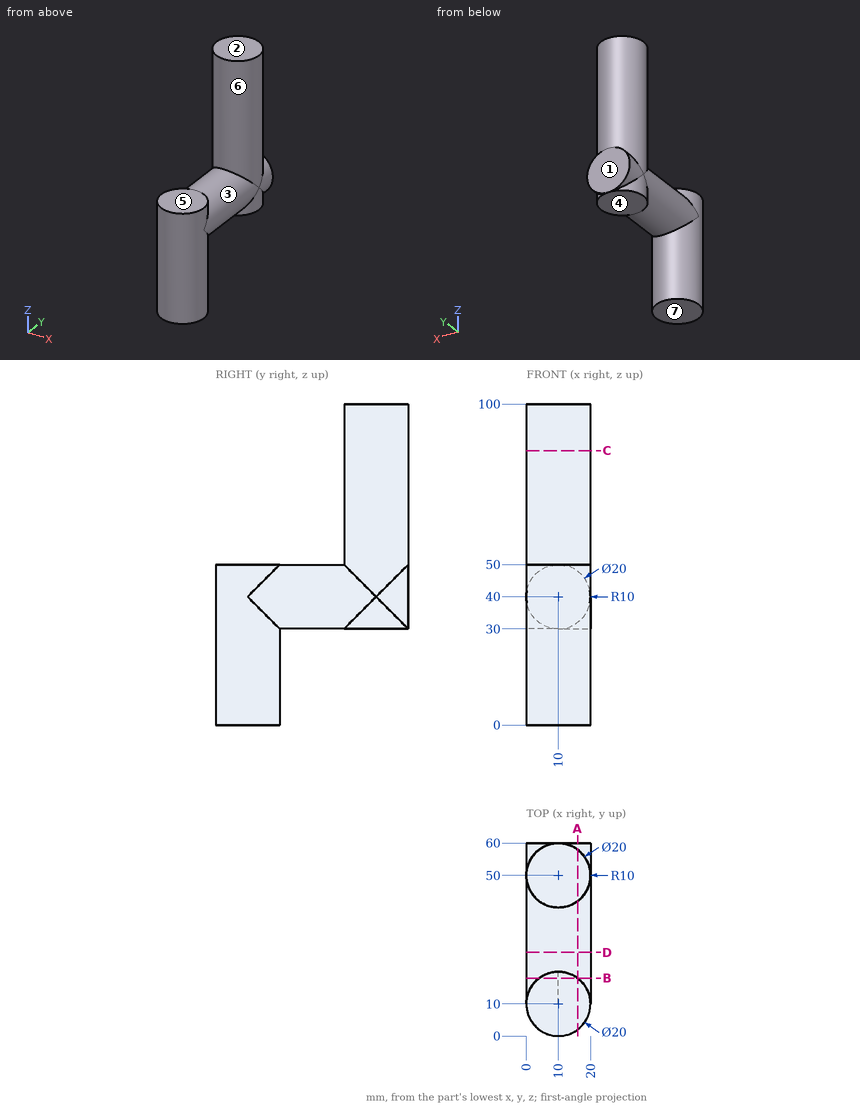
Check sheet for the drawn part. Datum: minimum x, y, z corner. Units: mm. A direction names the side the tool comes from. Coordinates: 2 decimals unless noted, no trailing zeros. Order: outer loops, then holes, each group sorted by start corner. A loop starts at its lowest first (then second) coordinate and runs counter-clockwise, first axis right, second up. Notation, with made-up numbers: M -16,-36 L 11,-36 A21 ccw 11,-14 Z; hole C -36,17 d3. An arc over 180 degrees is marked long. One line per item, written item: value. Start each with the question number.
Item 1: Mould release check, pull along Y, two halves, no side actions. Record for the marked faces 1, 2 and 3: released by +Y, released by -Y, zero draft, split by the parting line, or undercut.
Item 2: Sectioned sample at D-D (y = 26). Enter the section's corners in (x, z), then the cut area to 3 significant figures.
Item 3: Sectioned sample at C-C (z = 85.5). Enter the section's corners in (x, y).
Item 4: Sectioned sample at A-A (x = 16). Enter the section's corners in (y, z), then the cut area to 3 significant figures.
Item 5: Access from +Z, -Z, +X, -X, +Y, -Y to the whole of each face (thin tool, end or side, straight path). Record for the marked faces 4, 5, 6 and 7.
Item 6: Sectioned sample at B-B (y = 18). Enter the section's corners in (x, z).
Item 7: Scan lines: probe 1 along Z at (x, y) = (2.25, 45.5); probe 2 along Z at (x, y) = (14.75, 13.5); probe 3 along X at (y, z) = (4, 8). Record each from-to range of solid material in increasing order.
Item 8: Gauge pin test, flat ends, axial feed: pin 1 (6 mm diameter, centred on x = 11.5, y = 7, fed in from +Z); pin 2 (3 mm diameter, centred on x = 12, z = 69.5, fed in from -Y); pin 3 (1 mm diameter, centred on y = 47.5, z = 50.5, fed in from -X). Record the tip position at first contact, or that the pin passes through.
Conclusion:
1. face 1: released by +Y
1. face 2: zero draft
1. face 3: undercut
2. outline: C 10,40 d20
2. area: 314 mm^2
3. outline: C 10,50 d20
4. outline: M 2,0 L 18,0 L 18,32 L 42,32 L 42,30 L 58,30 L 58,32 L 60,32 L 60,48 L 58,48 L 58,100 L 42,100 L 42,48 L 18,48 L 18,50 L 2,50 Z
4. area: 2,340 mm^2
5. face 4: -Z, +X, -X, +Y
5. face 5: +Z, +X, -X, -Y
5. face 6: +Z
5. face 7: -Z, +X, -X, +Y, -Y
6. outline: M 4,0 L 16,0 L 16,32 A10 ccw 16,48 L 16,50 L 4,50 L 4,48 A10 ccw 4,32 Z
7. probe 1: z = 30 to 100
7. probe 2: z = 0 to 50
7. probe 3: x = 2 to 18
8. pin 1: stops at z = 50
8. pin 2: stops at y = 40.01
8. pin 3: stops at x = 0.2
